Build history of the part. All positions in model axes, mm. A direction names the side the tool comes from. Give positions to 0.01 mm unless a question says otherwise; leave off trailing zeros. Order: outer loops, then holes, each group sorted by start corner. A loop starts at its lowest first (then second) coordinate and runs counter-clockwise, first axis right, second up. Notation, with made-up numbers: (24, -33) -> (80, -33) arc R27 cw to (80, -11) -> close; hole circle Ø7 at (21.25, -17). An arc over 180 degrees is marked (long way). Use a Markdown table: item, result. Add a question column.
```python
from build123d import *

# Parameters (mm, degrees)
SKETCH1_W                = 20
SKETCH1_H                = 8
BOSS_EXTRUDE1_DEPTH      = 2
SKETCH2_W                = 15
SKETCH2_H                = 1
BOSS_EXTRUDE2_DEPTH      = 5
BOSS_EXTRUDE2_DEPTH_BACK = 2
SKETCH3_R                = 1.65
CUT_EXTRUDE1_DEPTH       = 3
FILLET1_R                = 1
FILLET2_R                = 2


with BuildPart() as part:
    # Sketch1 → Boss-Extrude1 (new body)
    with BuildSketch(Plane.XY):
        with Locations((10, 4)):
            Rectangle(SKETCH1_W, SKETCH1_H)
    extrude(amount=BOSS_EXTRUDE1_DEPTH)

    # Sketch2 → Boss-Extrude2 (add, two sides)
    with BuildSketch(Plane.XY.offset(2)) as boss_extrude2_sk:
        with Locations((22.5, 0.5)):
            Rectangle(SKETCH2_W, SKETCH2_H)
    extrude(amount=BOSS_EXTRUDE2_DEPTH)
    extrude(boss_extrude2_sk.sketch, amount=-BOSS_EXTRUDE2_DEPTH_BACK)

    # Sketch3 → Cut-Extrude1 (cut, through all)
    with BuildSketch(Plane.XY.offset(2)):
        with Locations((3.5, 4)):
            Circle(SKETCH3_R)
        with Locations((16.5, 4)):
            Circle(SKETCH3_R)
    extrude(amount=-CUT_EXTRUDE1_DEPTH, mode=Mode.SUBTRACT)

    # Fillet1
    fillet1_edges = [part.edges().sort_by_distance(p)[0] for p in [
        (20, 1, 1),
        (0, 8, 1),
        (20, 8, 1),
        (0, 0, 1),
    ]]
    fillet(fillet1_edges, radius=FILLET1_R)

    # Fillet2
    fillet2_edges = [part.edges().sort_by_distance(p)[0] for p in [
        (15, 0.5, 2),
    ]]
    fillet(fillet2_edges, radius=FILLET2_R)


solid = part.part
```
(1) Band-saw the part on C-C on y = 4. Give the cut face in (x, z).
(2) Pin check, flat tips, straight feed: pin 1 Ø4 at (x, z) = (4.5, 2.5) entering from +Y; pin 2 Ø2 at (x, z) = (22.5, 3.5) entering from +Y; pin 3 Ø3 at (x, y) = (9.5, 4.5) entering from +Z; pin 4 Ø1.6 at (y, z) = (5, 1) entering from +X. Stop position of each tip, or through.
(3) Band-saw the part on D-D on x = 18.5. Give the cut face in (y, z).
(4) Mould opens along X. For faces 4 (the face through (18.074, 4.496, 1.014)), 5 (the face through (22.4, 0.5, 7)), 6 (the face through (15, 0.5, 5.5)) say: released by +X, released by -X, zero draft, split by the parting line, or undercut.
(5) Band-saw the part on A-A on z = 1. Give the cut face in (x, y).
(6) Wall check: probe 1 along Y at (x, z) = (3.5, 1.4); probe 2 along X at (y, z) = (0.5, 5); probe 3 along Y at (x, z) = (18.25, 3.5). Give the ranges that are in metal, low to high.
(7) Tool access for faces 1 (the face through (20, 4, 1)), 2 (the face through (0, 4, 1)), 3 (the face through (23, 1, 3)): list every direction of +Z, -Z, +X, -X, +Y, -Y with a clear straight run to the whole face (end or side of a thin tool).
(8) Band-saw the part on B-B on x = 3.5. Give the cut face in (y, z), plus the area to 3 significant figures.
Response:
| question | item | result |
|---|---|---|
| 1 | outline | (0, 0) -> (1.85, 0) -> (1.85, 2) -> (0, 2) -> close; (5.15, 0) -> (14.85, 0) -> (14.85, 2) -> (5.15, 2) -> close; (18.15, 0) -> (20, 0) -> (20, 2) -> (18.15, 2) -> close |
| 2 | pin 1 | stops at y = 8 |
| 2 | pin 2 | stops at y = 1 |
| 2 | pin 3 | stops at z = 2 |
| 2 | pin 4 | stops at x = 20 |
| 3 | outline | (0, 0) -> (8, 0) -> (8, 2) -> (1, 2) -> (1, 7) -> (0, 7) -> close |
| 4 | face 4 | undercut |
| 4 | face 5 | zero draft |
| 4 | face 6 | released by -X |
| 5 | outline | (0, 1) arc R1 ccw to (1, 0) -> (30, 0) -> (30, 1) -> (21, 1) arc R1 cw to (20, 2) -> (20, 7) arc R1 ccw to (19, 8) -> (1, 8) arc R1 ccw to (0, 7) -> close; hole circle Ø3.3 at (3.5, 4); hole circle Ø3.3 at (16.5, 4) |
| 6 | probe 1 | y = 0 to 2.35, 5.65 to 8 |
| 6 | probe 2 | x = 15 to 30 |
| 6 | probe 3 | y = 0 to 1 |
| 7 | face 1 | +Z, -Z, +X, +Y |
| 7 | face 2 | +Z, -Z, -X, +Y, -Y |
| 7 | face 3 | +Z, +X, +Y |
| 8 | outline | (0, 0) -> (2.35, 0) -> (2.35, 2) -> (0, 2) -> close; (5.65, 0) -> (8, 0) -> (8, 2) -> (5.65, 2) -> close |
| 8 | area | 9.40 mm² |
